Can you work these out from the model? Positions are in its coordinate system, mm. Give positions to 0.01 mm unless a question says otherwise; leave off trailing zeros. Write each loop counter-clockwise with the first axis right and the second up, starting at its lowest first coordinate (ties: lowest second). Pieces come first, ordered by that corner, then holes.
1. If I drill on probe 1 along X at (y, z) = (176.5, 0.65); probe 2 along X at (y, z) = (85, 1.05); probe 3 along Y at (x, z) = (107.5, 2.1), over which ranges is the centre line in solid material (lowest first)?
2. Suppose I cut it at A-A (y = -85). Please give me the cut outline in (x, z), and give its area (3 significant figures).
3. Thinking about a two-plate mould opening in Y: for faces 1 (the flat face through (-200.21, 117.02, 1.48)), 2 (the flat face through (35.835, -247.964, 1.521)), 3 (the cylindrical face through (123.997, 39.048, 1.479)), which applies, pulls with the +Y half, pulls with the -Y half, needs draft (parallel to the pull), parting line crosses it, or undercut?
4. I'm going to push flat-ended pins straight in: pin 1 (1 mm diameter, centred on y = 36, z = 1.5, fed in from +X); pin 2 (0.9 mm diameter, centred on x = 137.5, z = 2, fed in from -Y); pin 3 (1 mm diameter, centred on y = 68.5, z = 2.5, fed in from +X). Where does each tip first touch, or does it pass through?
5. Suppose I cut it at B-B (y = -140.5). Please give me the cut outline in (x, z).
```python
from build123d import *

# Parameters (mm, degrees)
SKETCH_1_R          = 130
SKETCH_1_R_2        = 2
SKETCH_1_R_3        = 1.5
EXTRUDE_1_DEPTH     = 3
SKETCH_8_W          = 20
SKETCH_8_H          = 20
CUT_EXTRUDE_4_DEPTH = 4
FILLET_2_R          = 20
EXTRUDE_2_DEPTH     = 3
FILLET_3_R          = 20
SKETCH_10_R         = 4.5
CUT_EXTRUDE_5_DEPTH = 3


with BuildPart() as part:
    # 草图1 → 凸台-拉伸1 (new body)
    with BuildSketch(Plane.XY):
        Polygon((150.828607906, 202.550991214), (-150.828607906, 202.550991214), (-250.828607906, 29.345910457), (-100, -231.89690167), (100, -231.89690167), (250.828607906, 29.345910457), align=None)
        Circle(SKETCH_1_R, mode=Mode.SUBTRACT)
        with Locations((-104.711767321, 169.550991214)):
            Circle(SKETCH_1_R_2, mode=Mode.SUBTRACT)
        with Locations((-40.666940629, 169.550991214)):
            Circle(SKETCH_1_R_2, mode=Mode.SUBTRACT)
        with Locations((40.666940629, 169.550991214)):
            Circle(SKETCH_1_R_2, mode=Mode.SUBTRACT)
        with Locations((104.711767321, 169.550991214)):
            Circle(SKETCH_1_R_2, mode=Mode.SUBTRACT)
        with Locations((94.479581967, -175.458546182)):
            Circle(SKETCH_1_R_2, mode=Mode.SUBTRACT)
        with Locations((126.501995314, -119.994099286)):
            Circle(SKETCH_1_R_2, mode=Mode.SUBTRACT)
        with Locations((167.168935942, -49.556891928)):
            Circle(SKETCH_1_R_2, mode=Mode.SUBTRACT)
        with Locations((199.191349289, 5.907554968)):
            Circle(SKETCH_1_R_2, mode=Mode.SUBTRACT)
        with Locations((-199.191349288, 5.907554969)):
            Circle(SKETCH_1_R_2, mode=Mode.SUBTRACT)
        with Locations((-167.168935942, -49.556891928)):
            Circle(SKETCH_1_R_2, mode=Mode.SUBTRACT)
        with Locations((-126.501995314, -119.994099285)):
            Circle(SKETCH_1_R_2, mode=Mode.SUBTRACT)
        with Locations((-94.479581968, -175.458546182)):
            Circle(SKETCH_1_R_2, mode=Mode.SUBTRACT)
        with Locations((109.450202338, -207.52867108)):
            Circle(SKETCH_1_R_3, mode=Mode.SUBTRACT)
        with Locations((119.450202338, -190.208163004)):
            Circle(SKETCH_1_R_3, mode=Mode.SUBTRACT)
        with Locations((219.450202338, -17.003082247)):
            Circle(SKETCH_1_R_3, mode=Mode.SUBTRACT)
        with Locations((229.450202338, 0.317425828)):
            Circle(SKETCH_1_R_3, mode=Mode.SUBTRACT)
    extrude(amount=EXTRUDE_1_DEPTH)

    # 草图8 → 切除-拉伸4 (cut, through all)
    with BuildSketch(Plane.XY.offset(3)):
        with Locations((-132.5, 169.550991214)):
            Rectangle(SKETCH_8_W, SKETCH_8_H)
        Polygon((-209.42521159, 43.633124432), (-226.745719666, 33.633124432), (-216.745719666, 16.312616357), (-199.42521159, 26.312616357), align=None)
        Polygon((-84.245719666, -213.184115646), (-66.92521159, -203.184115646), (-76.92521159, -185.86360757), (-94.245719666, -195.86360757), align=None)
        Polygon((66.92521159, -203.184115646), (84.245719666, -213.184115646), (94.245719666, -195.86360757), (76.92521159, -185.86360757), align=None)
        Polygon((209.42521159, 43.633124432), (199.42521159, 26.312616357), (216.745719666, 16.312616357), (226.745719666, 33.633124432), align=None)
        with Locations((132.5, 169.550991214)):
            Rectangle(SKETCH_8_W, SKETCH_8_H)
    extrude(amount=-CUT_EXTRUDE_4_DEPTH, mode=Mode.SUBTRACT)

    # 圆角2
    fillet_2_edges = [part.edges().sort_by_distance(p)[0] for p in [
        (-150.828607906, 202.550991214, 1.5),
        (150.828607906, 202.550991214, 1.5),
        (250.828607906, 29.345910457, 1.5),
        (100, -231.89690167, 1.5),
        (-100, -231.89690167, 1.5),
        (-250.828607906, 29.345910457, 1.5),
    ]]
    fillet(fillet_2_edges, radius=FILLET_2_R)

    # 草图9 → 凸台-拉伸2 (add)
    with BuildSketch(Plane.XY.offset(3)):
        with BuildLine():
            Line((88.452994616, -231.89690167), (8.007023849, -231.89690167))
            Line((8.007023849, -231.89690167), (77.001755962, -271.731028829))
            Line((77.001755962, -271.731028829), (105.773502692, -221.89690167))
            ThreePointArc((105.773502692, -221.89690167), (98.452994616, -229.217409746), (88.452994616, -231.89690167))
        make_face()
        with BuildLine():
            ThreePointArc((245.055105214, 39.345910457), (247.734597138, 29.345910457), (245.055105214, 19.345910457))
            Line((245.055105214, 19.345910457), (273.826851943, 69.180037615))
            Line((273.826851943, 69.180037615), (204.83211983, 109.014164773))
            Line((204.83211983, 109.014164773), (245.055105214, 39.345910457))
        make_face()
    extrude(amount=-EXTRUDE_2_DEPTH)

    # 圆角3
    fillet_3_edges = [part.edges().sort_by_distance(p)[0] for p in [
        (77.001755962, -271.731028829, 1.5),
        (8.007023849, -231.89690167, 1.5),
        (204.83211983, 109.014164773, 1.5),
        (273.826851943, 69.180037615, 1.5),
    ]]
    fillet(fillet_3_edges, radius=FILLET_3_R)

    # 草图10 → 切除-拉伸5 (cut)
    with BuildSketch(Plane.XY.offset(3)):
        with Locations((-18.973410903, -201.605578304)):
            Circle(SKETCH_10_R)
        with Locations((38.182680295, -234.604662943)):
            Circle(SKETCH_10_R)
        with Locations((165.108846905, 117.23424499)):
            Circle(SKETCH_10_R)
        with Locations((222.264938103, 84.235160351)):
            Circle(SKETCH_10_R)
    extrude(amount=-CUT_EXTRUDE_5_DEPTH, mode=Mode.SUBTRACT)


solid = part.part
```
Checks:
1. probe 1: x = -165.87 to -142.5, -122.5 to 122.5, 142.5 to 165.87
1. probe 2: x = -218.7 to -98.36, 98.36 to 217.83, 226.7 to 246.43
1. probe 3: y = -218.91 to -73.1, 73.1 to 202.55
2. outline: (-184.81, 0) - (-98.36, 0) - (-98.36, 3) - (-184.81, 3) - close; (98.36, 0) - (184.81, 0) - (184.81, 3) - (98.36, 3) - close
2. area: 519 mm2
3. face 1: pulls with the +Y half
3. face 2: pulls with the -Y half
3. face 3: undercut
4. pin 1: stops at x = 254.96
4. pin 2: stops at y = -167.72
4. pin 3: stops at x = 265.54
5. outline: (-152.77, 0) - (152.77, 0) - (152.77, 3) - (-152.77, 3) - close
